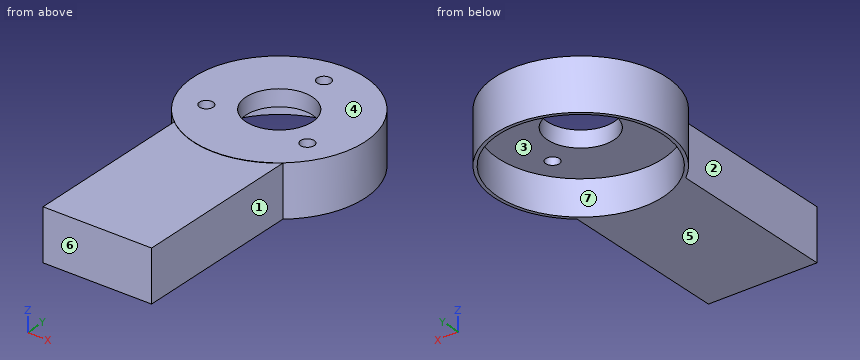
```python
from build123d import *

# Parameters (mm, degrees)
BOSS_EXTRUDE1_DEPTH      = 10
BOSS_EXTRUDE1_DEPTH_BACK = 3.242369731
SKETCH1_R                = 22
SKETCH1_R_2              = 1.75
SKETCH1_R_3              = 8.5
SKETCH2_W                = 27.907133148
SKETCH2_H                = 43.991238144
BOSS_EXTRUDE3_DEPTH      = 13.160474469
SKETCH3_R                = 21.15
CUT_EXTRUDE1_DEPTH       = 9


with BuildPart() as part:
    # Sketch1 → Boss-Extrude1 (new, two sides: drawn at the far end of the back side and taken through both)
    with BuildSketch(Plane.XY.offset(-BOSS_EXTRUDE1_DEPTH_BACK)):
        Circle(SKETCH1_R)
        with Locations((0, 15)):
            Circle(SKETCH1_R_2, mode=Mode.SUBTRACT)
        with Locations((12.990381057, -7.5)):
            Circle(SKETCH1_R_2, mode=Mode.SUBTRACT)
        with Locations((-12.990381057, -7.5)):
            Circle(SKETCH1_R_2, mode=Mode.SUBTRACT)
        Circle(SKETCH1_R_3, mode=Mode.SUBTRACT)
    extrude(amount=BOSS_EXTRUDE1_DEPTH + BOSS_EXTRUDE1_DEPTH_BACK)

    # Sketch2 → Boss-Extrude3 (add)
    with BuildSketch(Plane(origin=(0, 0, -3.242369731), x_dir=(-1, 0, 0), z_dir=(0, 0, -1))):
        with Locations((0, -39.004380928)):
            Rectangle(SKETCH2_W, SKETCH2_H)
    extrude(amount=-BOSS_EXTRUDE3_DEPTH)

    # Sketch3 → Cut-Extrude1 (cut)
    with BuildSketch(Plane(origin=(0, 0, -3.242369731), x_dir=(-1, 0, 0), z_dir=(0, 0, -1))):
        Circle(SKETCH3_R)
    extrude(amount=-CUT_EXTRUDE1_DEPTH, mode=Mode.SUBTRACT)


solid = part.part
```
Work out the finished part from the listing and answer in its coordinate system (mm). Face numbers are marked on the shaded views. A direction names the side the tool comes from. Give positions to 0.01 mm unless a question says otherwise; leave off trailing zeros. Write each loop counter-clockwise with the first axis right and the second up, starting at its lowest first coordinate (ties: lowest second). Pieces come first, ordered by that corner, then holes.
(1) The part is cut by section D-D on z = 1.75. Write down the section's boundary in (x, y), plus the area to 3 significant figures.
Final values:
outline: (-13.95, -61) - (13.95, -61) - (13.95, -17.01) arc R22 ccw (long way) to (-13.95, -17.01) - close; hole circle Ø42.3 at (0, 0)
area: 1,250 mm2
(2) The part is cut by section C-C on z = 8.5. Write down the section's boundary in (x, y).
Final values:
outline: (-13.95, -61) - (13.95, -61) - (13.95, -17.01) arc R22 ccw (long way) to (-13.95, -17.01) - close; hole circle Ø3.5 at (-12.99, -7.5); hole circle Ø17 at (0, 0); hole circle Ø3.5 at (0, 15); hole circle Ø3.5 at (12.99, -7.5)
(3) The part is cut by section B-B on x = -4. Write down the section's boundary in (y, z), plus the area to 3 significant figures.
Final values:
outline: (-61, -3.24) - (-20.77, -3.24) - (-20.77, 5.76) - (-7.5, 5.76) - (-7.5, 10) - (-21.63, 10) - (-21.63, 9.92) - (-61, 9.92) - close; (7.5, 5.76) - (20.77, 5.76) - (20.77, -3.24) - (21.63, -3.24) - (21.63, 10) - (7.5, 10) - close
area: 654 mm2
(4) Straight lines are drawn through the part: line 1 (Y direction, x = 0, z = 8.85); line 2 (X direction, y = -7.5, z = 7.4); line 3 (Z direction, x = 11.5, y = -22.5). For each, find the intervals that lie inside material, in ascending order.
Final values:
line 1: y = -61 to -8.5, 8.5 to 13.25, 16.75 to 22
line 2: x = -20.68 to -14.74, -11.24 to -4, 4 to 11.24, 14.74 to 20.68
line 3: z = -3.24 to 9.92
(5) The part is cut by section A-A on y = 0. Write down the section's boundary in (x, z).
Final values:
outline: (-22, -3.24) - (-21.15, -3.24) - (-21.15, 5.76) - (-8.5, 5.76) - (-8.5, 10) - (-22, 10) - close; (8.5, 5.76) - (21.15, 5.76) - (21.15, -3.24) - (22, -3.24) - (22, 10) - (8.5, 10) - close
(6) Which of the six approach directions +Z, -Z, +X, -X, +Y, -Y give full straight-line access (tool end or side, diameter ignored) to the marked faces 1, 2, 3 and 4?
Final values:
face 1: +Z, -Z, +X, -Y
face 2: +Z, -Z, -X, -Y
face 3: -Z
face 4: +Z, +X, -X, +Y, -Y
(7) Flat-ended cylindrical pins translate along their axes: pin 1 Ø6 at (x, z) = (-9.5, 3.5) entering from +Y; pin 2 Ø1.5 at (x, z) = (2, 3.5) entering from +Y; pin 3 Ø2 at (x, z) = (-9.5, -1.5) entering from +Y. Find the tip coordinate at first contact, or state that the pin passes through.
Final values:
pin 1: stops at y = 21.02
pin 2: stops at y = 21.96
pin 3: stops at y = 20.29
(8) The mould has two halves that part along Y. Classify the marked faces 5, 6 and 7: pulls with the +Y half, pulls with the -Y half, needs draft (parallel to the pull), parting line crosses it, or undercut.
Final values:
face 5: needs draft
face 6: pulls with the -Y half
face 7: undercut
